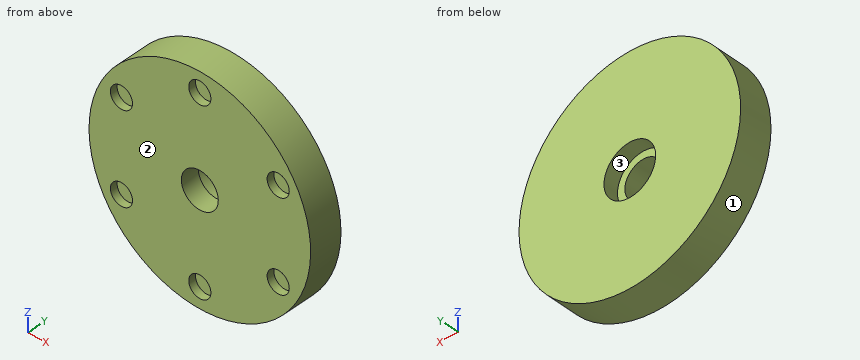
```python
from build123d import *

# Parameters (mm, degrees)
SKETCH1_R           = 38.1
SKETCH1_R_2         = 25.4
BOSS_EXTRUDE3_DEPTH = 6.35
SKETCH1_3_R         = 25.4
BOSS_EXTRUDE4_DEPTH = 6.35
SKETCH2_R           = 3.81
CUT_EXTRUDE1_DEPTH  = 2.54
SKETCH3_R           = 6.35
CUT_EXTRUDE2_DEPTH  = 55.254423783
SKETCH4_R           = 38.1
SKETCH4_R_2         = 8.89
BOSS_EXTRUDE5_DEPTH = 5.08


with BuildPart() as part:
    # Sketch1 → Boss-Extrude3 (new body)
    with BuildSketch(Plane(origin=(0, 0, 0), x_dir=(1, 0, 0), z_dir=(0, 1, 0))):
        with Locations(Location((0, 0, 0), (0, 0, 270))):
            Circle(SKETCH1_R)
        with Locations(Location((0, 0, 0), (0, 0, 270))):
            Circle(SKETCH1_R_2, mode=Mode.SUBTRACT)
    extrude(amount=BOSS_EXTRUDE3_DEPTH)

    # Sketch1_3 → Boss-Extrude4 (add)
    with BuildSketch(Plane(origin=(0, 0, 0), x_dir=(1, 0, 0), z_dir=(0, 1, 0))):
        Circle(SKETCH1_3_R)
    extrude(amount=BOSS_EXTRUDE4_DEPTH)

    # Sketch2 → Cut-Extrude1 (cut)
    with BuildSketch(Plane.XZ):
        with Locations(Location((0, 31.266403726, 0), (0, 0, 270))):
            Circle(SKETCH2_R)
        with Locations(Location((26.954852036, 15.704012647, 0), (0, 0, 270))):
            Circle(SKETCH2_R)
        with Locations(Location((26.954852036, -15.420769511, 0), (0, 0, 270))):
            Circle(SKETCH2_R)
        with Locations(Location((0, -30.98316059, 0), (0, 0, 270))):
            Circle(SKETCH2_R)
        with Locations(Location((-26.954852036, -15.420769511, 0), (0, 0, 270))):
            Circle(SKETCH2_R)
        with Locations(Location((-26.954852036, 15.704012647, 0), (0, 0, 270))):
            Circle(SKETCH2_R)
    extrude(amount=-CUT_EXTRUDE1_DEPTH, mode=Mode.SUBTRACT)

    # Sketch3 → Cut-Extrude2 (cut, through all)
    with BuildSketch(Plane(origin=(0, 6.35, 0), x_dir=(1, 0, 0), z_dir=(0, 1, 0))):
        with Locations(Location((0, 0, 0), (0, 0, 270))):
            Circle(SKETCH3_R)
    extrude(amount=-CUT_EXTRUDE2_DEPTH, mode=Mode.SUBTRACT)

    # Sketch4 → Boss-Extrude5 (add)
    with BuildSketch(Plane(origin=(0, 6.35, 0), x_dir=(1, 0, 0), z_dir=(0, 1, 0))):
        with Locations(Location((0, 0, 0), (0, 0, 270))):
            Circle(SKETCH4_R)
        with Locations(Location((0, 0, 0), (0, 0, 270))):
            Circle(SKETCH4_R_2, mode=Mode.SUBTRACT)
    extrude(amount=BOSS_EXTRUDE5_DEPTH)


solid = part.part
```
Geometry: final body of the model. Coordinates: model frame, mm. Face numbers are marked on the shaded views. Coordinates: 2 decimals unless noted, no trailing zeros. Order: outer loops, then holes, each group sorted by start corner. A loop starts at its lowest first (then second) coordinate and runs counter-clockwise, first axis right, second up. Notation, with made-up numbers: M -35.75,-19 L -25.75,-19 A20 ccw -25.75,20 Z; hole C 89.5,69 d7. An arc over 180 degrees is marked long. Answer in a Markdown table with one row per item. Add a question column.
Q1. Contact query for flat-ended pins moving along their axis: P1, Ø7, axis at x = 26.95, z = 15.7, coming from the -Y side; P2, Ø1.5, axis at x = 10, y = 2, coming from the +Z side; P3, Ø1, axis at x = 19, y = 10, coming from the -Z side. Output: stop coordinate, or through.
Q2. Section query C-C on y = 9.25. Return the cut outline in (x, z), and give its area (3 significant figures).
Q3. Section query A-A on x = 0. Return the cut outline in (y, z).
Q4. Line query: L1, parallel to X at y = 2.5, z = 0; L2, parallel to Y at x = -2.5, z = 7; L3, parallel to Z at x = -5.5, y = 8. Output: solid intervals per line, ascending.
Q5. Section query D-D on z = -8. Return the cut outline in (x, y).
Q6. Mould query, pull axis Z, two halves, no side actions, for the marked faces 1, 2 and 3. Classes: released by +Z, released by -Z, zero draft, split by the parting line, or undercut.
Q7. Section query B-B on z = 0. Return the cut outline in (x, y), and give its area (3 significant figures).
Completed:
| question | item | result |
|---|---|---|
| 1 | P1 | stops at y = 2.54 |
| 1 | P2 | stops at z = 36.96 |
| 1 | P3 | stops at z = -33.31 |
| 2 | outline | C 0,0 d76.2; hole C 0,0 d17.78 |
| 2 | area | 4,310 mm2 |
| 3 | outline | M 0,-38.1 L 11.43,-38.1 L 11.43,-8.89 L 6.35,-8.89 L 6.35,-6.35 L 0,-6.35 L 0,-27.17 L 2.54,-27.17 L 2.54,-34.79 L 0,-34.79 Z; M 0,6.35 L 6.35,6.35 L 6.35,8.89 L 11.43,8.89 L 11.43,38.1 L 0,38.1 L 0,35.08 L 2.54,35.08 L 2.54,27.46 L 0,27.46 Z |
| 4 | L1 | x = -38.1 to -6.35, 6.35 to 38.1 |
| 4 | L2 | y = 0 to 6.35 |
| 4 | L3 | z = -37.7 to -6.98, 6.98 to 37.7 |
| 5 | outline | M -37.25,0 L 37.25,0 L 37.25,11.43 L 3.88,11.43 L 3.88,6.35 L -3.88,6.35 L -3.88,11.43 L -37.25,11.43 Z |
| 6 | face 1 | split by the parting line |
| 6 | face 2 | zero draft |
| 6 | face 3 | undercut |
| 7 | outline | M -38.1,0 L -6.35,0 L -6.35,6.35 L -8.89,6.35 L -8.89,11.43 L -38.1,11.43 Z; M 6.35,0 L 38.1,0 L 38.1,11.43 L 8.89,11.43 L 8.89,6.35 L 6.35,6.35 Z |
| 7 | area | 700 mm2 |
